Here's the drawing with two shaded views (mm, measured from the low corner). I have some questions. A direction names the side the tool comes from. Coordinates: 2 decimals unless noted, no trailing zeros. Write each loop counter-clockwise with the first axis right and the second up, starting at its lowest first coordinate (ties: lowest second). Pieces come first, ordered by that corner, then holes.
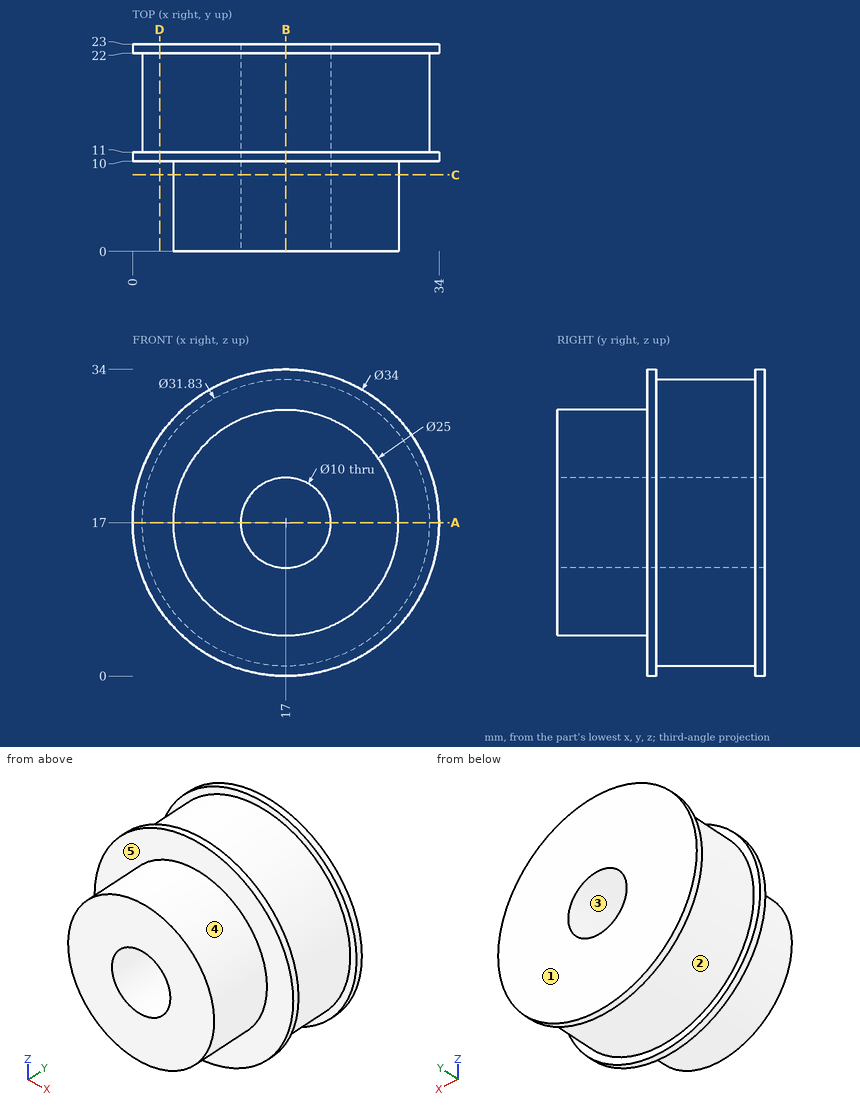
1. I want a section at B-B on x = 17. Please give me the cut outline in (y, z) (3 decimals), plus the area to 3 significant figures.
Verdict:
outline: (0, 4.5) - (10, 4.5) - (10, 0) - (11, 0) - (11, 1.085) - (22, 1.085) - (22, 0) - (23, 0) - (23, 12) - (0, 12) - close; (0, 22) - (23, 22) - (23, 34) - (22, 34) - (22, 32.915) - (11, 32.915) - (11, 34) - (10, 34) - (10, 29.5) - (0, 29.5) - close
area: 438 mm2
2. I want a section at A-A on z = 17. Please give me the cut outline in (x, y) (3 decimals), plus the area to 3 significant figures.
Verdict:
outline: (0, 10) - (4.5, 10) - (4.5, 0) - (12, 0) - (12, 23) - (0, 23) - (0, 22) - (1.085, 22) - (1.085, 11) - (0, 11) - close; (22, 0) - (29.5, 0) - (29.5, 10) - (34, 10) - (34, 11) - (32.915, 11) - (32.915, 22) - (34, 22) - (34, 23) - (22, 23) - close
area: 438 mm2
3. I want a section at D-D on x = 3. Please give me the cut outline in (y, z).
Verdict:
outline: (10, 7.36) - (11, 7.36) - (11, 9.43) - (22, 9.43) - (22, 7.36) - (23, 7.36) - (23, 26.64) - (22, 26.64) - (22, 24.57) - (11, 24.57) - (11, 26.64) - (10, 26.64) - close
4. I want a section at C-C on y = 8.5. Please give me the cut outline in (x, z).
Verdict:
outline: circle Ø25 at (17, 17); hole circle Ø10 at (17, 17)
5. Please list where these lines run through material, in increasing order: line 1 along X through (y, z) = (5, 17); line 2 along X through (y, z) = (14, 17) (3 decimals); line 3 along Y through (x, z) = (11.5, 31).
Verdict:
line 1: x = 4.5 to 12, 22 to 29.5
line 2: x = 1.085 to 12, 22 to 32.915
line 3: y = 10 to 23
6. For pin 1 (17 mm diameter, centred on x = 19.5, z = 8.5, fed in from -Y); pin 2 (5 mm diameter, centred on y = 11, z = 30.5, fed in from +X); pin 3 (2 mm diameter, centred on y = 8.5, z = 24.5, fed in from -X); pin 4 (8 mm diameter, centred on x = 24, y = 5, fed in from -Z), each with a flat end and sliding along its axis, tell me the tip position at first contact or that it passes through.
Verdict:
pin 1: stops at y = 0
pin 2: stops at x = 29.96
pin 3: stops at x = 6.32
pin 4: stops at z = 4.87
7. If we mould it in two halves opening along Z, with no side actions, what happens to the marked faces 3, 4 and 5? For each: pulls with the +Z half, pulls with the -Z half, needs draft (parallel to the pull), parting line crosses it, or undercut.
Verdict:
face 3: undercut
face 4: parting line crosses it
face 5: needs draft
8. On a 3-axis mill with a long thin cutter (end or side, diameter ignored), from which of +Z, -Z, +X, -X, +Y, -Y can I reach the whole of each face in a straight line? I mean the marked faces 1 and 2. Say none if no direction works.
Verdict:
face 1: +Z, -Z, +X, -X, +Y
face 2: none
